Geometry check sheet. Reference: the model listing, model coordinates, mm. A direction names the side the tool comes from. Coordinates: 2 decimals unless noted, no trailing zeros. Order: outer loops, then holes, each group sorted by start corner. A loop starts at its lowest first (then second) coordinate and runs counter-clockwise, first axis right, second up.
```python
from build123d import *

# Parameters (mm, degrees)
F1_DEPTH = 45
F2_R     = 2


with BuildPart() as f1:
    # F0 (on Top) → F1 (new body)
    with BuildSketch(Plane.XY):
        Polygon((0, 45), (0, 0), (31.819805, -31.819805), (63.63961, 0), (45, 18.63961), (45, 45), align=None)
    extrude(amount=F1_DEPTH)

    # F2
    f2_edges = [f1.edges().sort_by_distance(p)[0] for p in [
        (54.319805, 9.319805, 0),
        (45, 31.819805, 0),
        (15.909903, -15.909903, 0),
        (0, 22.5, 0),
        (54.319805, 9.319805, 45),
        (45, 31.819805, 45),
        (0, 22.5, 45),
        (15.909903, -15.909903, 45),
    ]]
    fillet(f2_edges, radius=F2_R)


solid = f1.part
```
Item 1: Sectioned sample at B-B (z = 38). Record the cut outline in (x, y), and give its area (3 significant figures).
Item 2: Depth check by flat-ended pin: P1, Ø21, axis at y = 33.5, z = 24.5, coming from the +X side; P2, Ø1.5, axis at y = -21.5, z = 9.5, coming from the +X side; P3, Ø1.5, axis at y = 8, z = 25, coming from the +X side. Enter the tip coordinate at first touch or a pass-through.
Item 3: Sectioned sample at A-A (y = 28). Record the cut outline in (x, z).
Item 4: Tool access check on faces 1 (the face through (44.43, 31.6, 0.6)), 2 (the face through (16.54, -15.73, 44.4)), 3 (the face through (47.51, -16.13, 22.18)), 4 (the face through (44.43, 31.6, 44.4)), 5 (the face through (45, 32, 22)). Record the directions out of +Z, -Z, +X, -X, +Y, -Y that give a thin tool (end or side, any length) a straight path to the whole face; none if there is none.
Item 5: Thickness scan on line 1 along X through (y, z) = (39.5, 23); line 2 along X through (y, z) = (3, 31). Record the ranges inside material, lowest first.
Geometry check:
1. outline: (0, 0) - (31.82, -31.82) - (63.64, 0) - (45, 18.64) - (45, 45) - (0, 45) - close
1. area: 3,210 mm2
2. P1: stops at x = 45
2. P2: stops at x = 42.89
2. P3: stops at x = 56.39
3. outline: (0, 2) arc R2 ccw to (2, 0) - (43, 0) arc R2 ccw to (45, 2) - (45, 43) arc R2 ccw to (43, 45) - (2, 45) arc R2 ccw to (0, 43) - close
4. face 1: -Z, +X, +Y
4. face 2: +Z, -X, -Y
4. face 3: +Z, -Z, +X, -Y
4. face 4: +Z, +X, +Y
4. face 5: +Z, -Z, +X, +Y
5. line 1: x = 0 to 45
5. line 2: x = 0 to 60.64
